from build123d import *

# Parameters (mm, degrees)
F0_R     = 12.1158
F0_R_2   = 4.7498
F0_R_3   = 11.049
F1_DEPTH = 8.8138
F2_R     = 7.62


# Not quite as in the source:
# - ends of sketch curves that miss each other by under 0.0002 mm in the source are joined


with BuildPart() as f1:
    # F0 (on Top) → F1 (new body)
    with BuildSketch(Plane.XY):
        with BuildLine():
            ThreePointArc((22.4249021167, -33.2598383611), (42.5511926564, -11.3994547245), (48.2521252698, 17.762906479))
            ThreePointArc((48.2521252698, 17.762906479), (39.4932996014, 26.5789641765), (27.0699823404, 26.8969085886))
            Line((27.0699823404, 26.8969085886), (-8.0010006819, 13.8581388051))
            ThreePointArc((-8.0010006819, 13.8581388051), (-10.1044657967, 14.3898463988), (-10.3558611613, 16.5448588871))
            ThreePointArc((-10.3558611613, 16.5448588871), (1.2618519363, 29.6731834096), (17.5914130917, 36.0504551503))
            ThreePointArc((17.5914130917, 36.0504551503), (-11.4033797439, 42.5501422233), (-39.5091916872, 32.90611409))
            ThreePointArc((-39.5091916872, 32.90611409), (-42.7647087802, 20.9127197051), (-36.8283980876, 9.9948391518))
            Line((-36.8283980876, 9.9948391518), (-8.0010006819, -13.8581382646))
            ThreePointArc((-8.0010006819, -13.8581382646), (-7.409740408, -15.9456462868), (-9.1503382861, -17.2408673032))
            ThreePointArc((-9.1503382861, -17.2408673032), (-26.3286573805, -13.743794888), (-40.0163172925, -2.7906159651))
            ThreePointArc((-40.0163172925, -2.7906159651), (-31.1478149966, -31.1506866748), (-8.7429356667, -50.669019745))
            ThreePointArc((-8.7429356667, -50.669019745), (3.2714070948, -47.4916830576), (9.7584136631, -36.8917469163))
            Line((9.7584136631, -36.8917469163), (16.0019992774, 2.702e-07))
            ThreePointArc((16.0019992774, 2.702e-07), (17.514204114, 1.5558007108), (19.5061973633, 0.6960092401))
            ThreePointArc((19.5061973633, 0.6960092401), (25.0668033601, -15.9293876975), (22.4249021167, -33.2598383611))
        make_face()
        with Locations((-4.651045185, -34.7045873419)):
            Circle(F0_R, mode=Mode.SUBTRACT)
        with Locations((-24.3930550349, -25.1201008156)):
            Circle(F0_R_2, mode=Mode.SUBTRACT)
        with Locations((33.9511726837, -8.5649542264)):
            Circle(F0_R_2, mode=Mode.SUBTRACT)
        Circle(F0_R_3, mode=Mode.SUBTRACT)
        with Locations((-27.7295329099, 21.3802167818)):
            Circle(F0_R, mode=Mode.SUBTRACT)
        with Locations((-9.5581186852, 33.6850558475)):
            Circle(F0_R_2, mode=Mode.SUBTRACT)
        with Locations((32.3805760108, 13.3243713841)):
            Circle(F0_R, mode=Mode.SUBTRACT)
    extrude(amount=F1_DEPTH)

    # F2
    f2_edges = [f1.edges().sort_by_distance(p)[0] for p in [
        (-39.509192, 32.906114, 4.4069),
        (48.252125, 17.762906, 4.4069),
        (-8.742936, -50.66902, 4.4069),
    ]]
    fillet(f2_edges, radius=F2_R)


solid = f1.part
Design review of the part built by this model. Coordinates are the model's own, in mm. A direction names the side the tool comes from. Give positions to 0.01 mm unless a question says otherwise; leave off trailing zeros. Order: outer loops, then holes, each group sorted by start corner. A loop starts at its lowest first (then second) coordinate and runs counter-clockwise, first axis right, second up. Notation, with made-up numbers: (46, 69) - (92, 69) arc R28 cw to (92, 88) - close; hole circle Ø11 at (60.25, 32.5). An arc over 180 degrees is marked (long way). Write item = value, one per line. Start each with the question number.
Q1. To check wall thickness, follow L1, parallel to X at y = 31, z = 2.25; L2, parallel to Y at x = -4, z = 2.25; L3, parallel to Y at x = 34.5, z = 5.5. State the ranges of each line that lie inside material, in increasing order. Write a range as from..to.
Q2. Clearance check with flat-ended pins moving along their axes: pin 1 Ø19.5 at (x, y) = (-27.73, 21.38) entering from +Z; pin 2 Ø4 at (y, z) = (-24.5, 2.5) entering from -X; pin 3 Ø1 at (y, z) = (-9.5, 5) entering from +X; pin 4 Ø3 at (y, z) = (0, 5) entering from -X. State where each tip first meets the part, or that it passes through.
Q3. Mouldability with a two-part tool opening along X and no side actions: class faces 1 (the face through (38.715, 26.892, 4.345)), 2 (the face through (12, -3, 0)), 3 (the face through (-10.198, 42.603, 4.345)) as released by +X, released by -X, zero draft, split by the parting line, or undercut.
Q4. We need section A-A on x = 0. State the section outline as (y, z) points.
Q5. Tool access review of faces 4 (the face through (12, -3, 8.814)), 5 (the face through (9.78, 20.47, 4.35)): name each direction out of +Z, -Z, +X, -X, +Y, -Y from which nothing blocks a thin tool from reaching the whole face with its end or side.
Q6. We need section B-B on z = 3. State how many separate pieces and enclosed holes the cut face has, plus the area to 3 significant figures.
Working result:
q1.L1 = -40.75..-35.1, -20.36..-13.48, -5.64..3.3
q1.L2 = -50.58..-46.8, -22.61..-10.3, 10.3..15.35, 25.23..42.46
q1.L3 = -23.18..-13.28, -3.85..1.4, 25.25..27.86
q2.pin_1 = through
q2.pin_2 = -35.75
q2.pin_3 = 43.69
q2.pin_4 = -26.56
q3.face_1 = undercut
q3.face_2 = zero draft
q3.face_3 = split by the parting line
q4.outline = (-49.39, 0) - (-45.89, 0) - (-45.89, 8.81) - (-49.39, 8.81) - close; (-23.52, 0) - (-11.05, 0) - (-11.05, 8.81) - (-23.52, 8.81) - close; (11.05, 0) - (16.83, 0) - (16.83, 8.81) - (11.05, 8.81) - close; (28.75, 0) - (41.98, 0) - (41.98, 8.81) - (28.75, 8.81) - close
q5.face_4 = +Z, +X, -X, +Y, -Y
q5.face_5 = +Z, -Z
q6.separate_pieces = 1
q6.enclosed_holes = 7
q6.area = 3,020 mm²
